```python
from build123d import *

# Parameters (mm, degrees)
PAD001_DEPTH = 10
SKETCH_R     = 17
PAD_DEPTH    = 10
SKETCH001_R  = 14.75
POCKET_DEPTH = 10


with BuildPart() as adapter_ring_cutout:
    # Sketch002 → Pad001 (new body)
    with BuildSketch(Plane.XY):
        Polygon((-3, 17), (3, 17), (2, 14), (-2, 14), align=None)
    extrude(amount=PAD001_DEPTH)


with BuildPart() as cut:
    # Sketch → Pad (new body)
    with BuildSketch(Plane.XY):
        Circle(SKETCH_R)
    extrude(amount=PAD_DEPTH)

    # Sketch001 (on Face3 of Pad) → Pocket (cut)
    with BuildSketch(Plane.XY.offset(10)):
        Circle(SKETCH001_R)
    extrude(amount=-POCKET_DEPTH, mode=Mode.SUBTRACT)

    # Cut: cut adapter ring cutout
    add(adapter_ring_cutout.part, mode=Mode.SUBTRACT)


solid = cut.part
```
CAD build for the part. Positions are in the model's coordinates, mm. A direction names the side the tool comes from. Round coordinates to 2 decimals unless told otherwise and drop trailing zeros. Order: outer loops, then holes, each group sorted by start corner. A loop starts at its lowest first (then second) coordinate and runs counter-clockwise, first axis right, second up. Notation, with made-up numbers: (54.25, 37.25) -> (92.25, 37.25) arc R35 cw to (92.25, 71.25) -> close; hole circle Ø7 at (19, 83). An arc over 180 degrees is marked (long way). Write item = value, one per line.
(1) Cut at A-A (y = 0). Write the cut outline in (x, z).
Answers follow:
outline = (-17, 0) -> (-14.75, 0) -> (-14.75, 10) -> (-17, 10) -> close; (14.75, 0) -> (17, 0) -> (17, 10) -> (14.75, 10) -> close
(2) Pull direction X, two halves, no side cores. Call faces 3 (the flat face through (-2.55, 15.65, 4.93)), 4 (the flat face through (0, -15, 10)), 5 (the cylindrical face through (-0.706, -16.985, 4.93)): +X half, -X half, draft (parallel to the pull), parting line (faces both ways), or undercut.
Answers follow:
face_3 = undercut
face_4 = draft
face_5 = parting line
(3) Flat gauge pins, fed straight in: P1, Ø4, axis at x = 11, z = 6.5, coming from the -Y side; P2, Ø3, axis at y = 5.5, z = 4.5, coming from the -X side; P3, Ø1, axis at x = -5, z = 3, coming from the -Y side; P4, Ø1.5, axis at x = 2.5, z = 8.5, coming from the +Y side. Where does each tip first touch, or does it go through?
Answers follow:
P1 = -14.42
P2 = -16.52
P3 = -16.39
P4 = 16.75
(4) Cut at C-C (x = 0). Write the cut outline in (y, z).
Answers follow:
outline = (-17, 0) -> (-14.75, 0) -> (-14.75, 10) -> (-17, 10) -> close
(5) Drill centre lines: L1, parallel to X at y = 0, z = 2.5; L2, parallel to Y at x = 13, z = 2; L3, parallel to Y at x = 0, z = 5.5. Where is each one in solid material? Low to high.
Answers follow:
L1 = -17 to -14.75, 14.75 to 17
L2 = -10.95 to -6.97, 6.97 to 10.95
L3 = -17 to -14.75
(6) 3-axis set-ups, long thin cutter, end or side, ignore diameter. For faces 1 (the flat face through (2.56, 15.68, 4.93)), 2 (the flat face through (0, -15, 0)): which of +Z, -Z, +X, -X, +Y, -Y reach the whole face in a straight line?
Answers follow:
face_1 = +Z, -Z, +Y
face_2 = -Z, +X, -X, +Y, -Y
(7) Cut at B-B (x = -5.5). Write the cut outline in (y, z).
Answers follow:
outline = (-16.09, 0) -> (-13.69, 0) -> (-13.69, 10) -> (-16.09, 10) -> close; (13.69, 0) -> (16.09, 0) -> (16.09, 10) -> (13.69, 10) -> close
